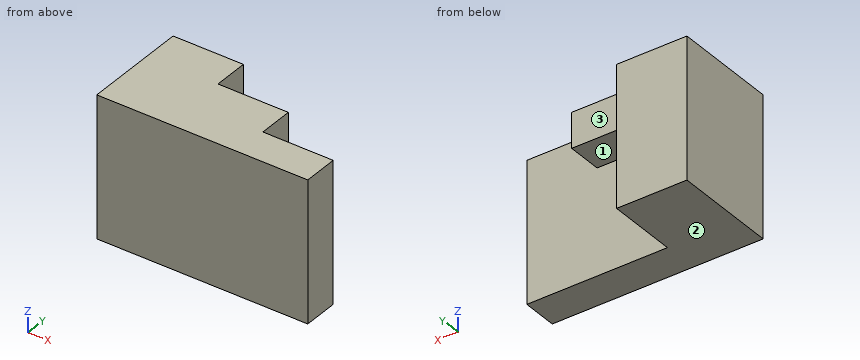
from build123d import *

# Parameters (mm, degrees)
F1_DEPTH = 40
F2_W     = 20
F2_H     = 10
F3_DEPTH = 10


with BuildPart() as f1:
    # F0 (on Top) → F1 (new body)
    with BuildSketch(Plane.XY):
        Polygon((0, 30), (0, 0), (60, 0), (60, 10), (20, 10), (20, 30), align=None)
    extrude(amount=F1_DEPTH)

    # F2 (on face) → F3 (join)
    with BuildSketch(Plane(origin=(0, 10, 0), x_dir=(-1, 0, 0), z_dir=(0, 1, 0))):
        with Locations((-30, 35)):
            Rectangle(F2_W, F2_H)
    extrude(amount=F3_DEPTH)


solid = f1.part
Part model, mm, in its own coordinate system. Face numbers are marked on the shaded views. A direction names the side the tool comes from. Coordinates: 2 decimals unless noted, no trailing zeros. Order: outer loops, then holes, each group sorted by start corner. A loop starts at its lowest first (then second) coordinate and runs counter-clockwise, first axis right, second up. Notation, with made-up numbers: M -21.75,-4 L -9.75,-4 A26 ccw -9.75,33 Z; hole C 83.5,39 d9. An arc over 180 degrees is marked long. Use a Markdown table: item, result.
(1) Probe L1, parallel to X at y = 15.5, z = 20; L2, parallel to X at y = 14, z = 36.5; L3, parallel to Y at x = 56, z = 35. List the from-to ranges inside material, lowest first.
A:
| item | result |
|---|---|
| L1 | x = 0 to 20 |
| L2 | x = 0 to 40 |
| L3 | y = 0 to 10 |
(2) Cut at D-D on z = 34. Write the cut outline in (x, y), then the cut area to 3 significant figures.
A:
| item | result |
|---|---|
| outline | M 0,0 L 60,0 L 60,10 L 40,10 L 40,20 L 20,20 L 20,30 L 0,30 Z |
| area | 1,200 mm^2 |
(3) Cut at B-B on z = 28. Write the cut outline in (x, y).
A:
| item | result |
|---|---|
| outline | M 0,0 L 60,0 L 60,10 L 20,10 L 20,30 L 0,30 Z |
(4) Cut at C-C on y = 25.5. Write the cut outline in (x, z).
A:
| item | result |
|---|---|
| outline | M 0,0 L 20,0 L 20,40 L 0,40 Z |
(5) Flat gauge pins, fed straight in: pin 1 (5 mm diameter, centred on x = 30, z = 33.5, fed in from +Y); pin 2 (3 mm diameter, centred on y = 15, z = 34.5, fed in from +X); pin 3 (8 mm diameter, centred on x = 26, y = 15, fed in from -Z). Where does each tip first touch, or does it go through?
A:
| item | result |
|---|---|
| pin 1 | stops at y = 20 |
| pin 2 | stops at x = 40 |
| pin 3 | stops at z = 30 |
(6) Tool access for the marked faces 1, 2 and 3: list every direction of +Z, -Z, +X, -X, +Y, -Y with a clear straight run to the whole face (end or side of a thin tool).
A:
| item | result |
|---|---|
| face 1 | -Z, +X, +Y |
| face 2 | -Z, +X, -X, +Y, -Y |
| face 3 | +Z, -Z, +X, +Y |
(7) Cut at A-A on x = 29. Write the cut outline in (y, z).
A:
| item | result |
|---|---|
| outline | M 0,0 L 10,0 L 10,30 L 20,30 L 20,40 L 0,40 Z |
